from build123d import *

# Parameters (mm, degrees)
BOSS_EXTRUDE1_DEPTH = 12.7
CHAMFER1_SIZE       = 10.16
CHAMFER1_SIZE2      = 3.69793758


with BuildPart() as part:
    # Sketch1 → Boss-Extrude1 (new body)
    with BuildSketch(Plane(origin=(0, 0, 0), x_dir=(1, 0, 0), z_dir=(0, 1, 0))):
        Polygon((0, 0), (63.5, 0), (63.5, 68.58), (50.8, 68.58), (50.8, 50.8), (12.7, 50.8), (12.7, 68.58), (0, 68.58), align=None)
    extrude(amount=BOSS_EXTRUDE1_DEPTH)

    # Chamfer1
    chamfer1_edges = [part.edges().sort_by_distance(p)[0] for p in [
        (0, 0, -34.29),
        (63.5, 0, -34.29),
    ]]
    chamfer1_side = [part.faces().sort_by_distance(p)[0] for p in [
        (31.75, 0, -29.611052632),
    ]]
    chamfer(chamfer1_edges, length=CHAMFER1_SIZE, length2=CHAMFER1_SIZE2, reference=chamfer1_side[0])


solid = part.part
Could you check a few things on this model? Use its own coordinates, in mm. A direction names the side the tool comes from. Give positions to 0.01 mm unless a question says otherwise; leave off trailing zeros. Loops run counter-clockwise (first coordinate to the right, second up) from the corner with the lowest first, then second, coordinate; pieces in that order, holes last. Notation, with made-up numbers: (21, 82) -> (66, 82) arc R12 ccw to (66, 86) -> close; hole circle Ø1 at (65, -1.5). An arc over 180 degrees is marked (long way). Answer as CSV lines item,"result". Start each with the question number.
(1) I need wall thicknesses on probe 1 along X at (y, z) = (7.25, -58.5); probe 2 along Z at (x, y) = (38, 9); probe 3 along Y at (x, z) = (55, -17). Which ranges of each line are inside material? Lowest first, please.
(2) If we section it at C-C on z = -11: Write out the boundary of the cut face in (x, y).
(3) I'm going to push a flat-ended pin straight in: pin 1 Ø6.5 at (x, y) = (41, 8) entering from -Z. Where does the tip first touch, or does it pass through?
(4) If we section it at D-D on x = 14: Write out the boundary of the cut face in (y, z).
(5) If we section it at A-A on z = -64: Write out the boundary of the cut face in (x, y).
(6) We'd pull the mould along X, two halves only. Please class faces 1 (the flat face through (57, 6, -68.58)), 2 (the flat face through (63.5, 8, -34)), 3 (the flat face through (50.8, 6, -60)), 4 (the flat face through (12.7, 6, -60)): released by +X, released by -X, zero draft, split by the parting line, or undercut.
(7) Which directions (+Z, -Z, +X, -X, +Y, -Y) give clear straight access to the entire face, cutting with the end or side of a thin tool? Please do faces 5 (the flat face through (31, 6, 0)), 6 (the flat face through (32, 6, -50.8)).
(8) If we section it at B-B on y = 9.5: Write out the boundary of the cut face in (x, z).
Computed:
1,probe 1,"x = 0 to 12.7, 50.8 to 63.5"
1,probe 2,"z = -50.8 to 0"
1,probe 3,"y = 0.6 to 12.7"
2,outline,"(0, 3.7) -> (10.16, 0) -> (53.34, 0) -> (63.5, 3.7) -> (63.5, 12.7) -> (0, 12.7) -> close"
3,pin 1,"stops at z = -50.8"
4,outline,"(0, -50.8) -> (12.7, -50.8) -> (12.7, 0) -> (0, 0) -> close"
5,outline,"(0, 3.7) -> (10.16, 0) -> (12.7, 0) -> (12.7, 12.7) -> (0, 12.7) -> close; (50.8, 0) -> (53.34, 0) -> (63.5, 3.7) -> (63.5, 12.7) -> (50.8, 12.7) -> close"
6,face 1,"zero draft"
6,face 2,"released by +X"
6,face 3,"undercut"
6,face 4,"undercut"
7,face 5,"+Z, +X, -X, +Y, -Y"
7,face 6,"-Z, +Y, -Y"
8,outline,"(0, -68.58) -> (12.7, -68.58) -> (12.7, -50.8) -> (50.8, -50.8) -> (50.8, -68.58) -> (63.5, -68.58) -> (63.5, 0) -> (0, 0) -> close"
